CAD build for the part. Positions are in the model's coordinates, mm. A direction names the side the tool comes from. Round coordinates to 2 decimals unless told otherwise and drop trailing zeros. Loops run counter-clockwise (first coordinate to the right, second up) from the corner with the lowest first, then second, coordinate; pieces in that order, holes last. Notation, with made-up numbers: (11.5, -23.75) - (45.5, -23.75) arc R20 cw to (45.5, 5.25) - close; hole circle Ø3 at (58, 42.25). An arc over 180 degrees is marked (long way). One line per question, with ' | ' between items.
Autodesk Inventor part; units mm, degrees
ref_plane "dia1_XY" through (0, 3.175, 0) normal (1, 0, 0) x (0, 0, -1)
ref_plane "dia1_YZ" through (0, 3.175, 0) normal (0, 0, -1) x (0, 1, 0)
ref_plane "dia1_ZX" through (0, 3.175, 0) normal (0, 1, 0) x (1, 0, 0)
sketch "Sketch_1" plane through (0, 0, 0) normal (0, 0, 1) x (1, 0, 0)
  line L0 (67.5386, 0) -> (0, 0)
  line L1 (0, 0) -> (0, 3.175)
  line L2 (0, 3.175) -> (47.625, 3.175)
  line L3 (47.625, 3.175) -> (47.625, 9.6202)
  line L4 (47.625, 9.6202) -> (67.5386, 9.6202)
  line L5 (67.5386, 9.6202) -> (67.5386, 0)
  line L6 (67.5386, 0) -> (0, 0)
revolve "Revolution1" add sketch "Sketch_1" angle 360 about axis through (67.5386, 0, 0) along (1, 0, 0)
sketch "Sketch_3" plane through (0, 0, 0) normal (0, 0, 1) x (1, 0, 0)
  line L0 (0, 0) -> (-12.7, 0)
  line L1 (-12.7, 0) -> (-12.7, 2.634)
  line L2 (-12.7, 2.634) -> (-12.159, 3.175)
  line L3 (-12.159, 3.175) -> (0, 3.175)
  line L4 (0, 3.175) -> (0, 0)
  line L5 (0, 0) -> (-12.7, 0)
revolve "Revolution2" add sketch "Sketch_3" angle 360 about axis through (0, 0, 0) along (1, 0, 0)
sketch "Sketch_30" plane through (0, 0, 0) normal (0, 0, 1) x (1, 0, 0)
  line L0 (0, 0) -> (-0.254, 0)
  line L1 (-0.254, 2.921) -> (0, 2.921)
  line L2 (0, 2.921) -> (0, 3.429)
  line L3 (0, 3.429) -> (-0.254, 3.429)
  line L4 (-0.254, 3.429) -> (-0.254, 2.921)
revolve "Revolution3" cut sketch "Sketch_30" angle 360 about axis through (0, 0, 0) along (1, 0, 0)
ref_plane "dia1_XY" through (0, 3.175, 0) normal (1, 0, 0) x (0, 0, -1)
ref_plane "dia1_YZ" through (0, 3.175, 0) normal (0, 0, -1) x (0, 1, 0)
ref_plane "dia1_ZX" through (0, 3.175, 0) normal (0, 1, 0) x (1, 0, 0)
ref_plane "dia12_XY" through (0, 0, 10.2235) normal (1, 0, 0) x (0, 0, -1)
ref_plane "dia12_YZ" through (0, 0, 10.2235) normal (0, 0, -1) x (0, 1, 0)
ref_plane "dia12_ZX" through (0, 0, 10.2235) normal (0, 1, 0) x (1, 0, 0)
ref_plane "dia2_XY" through (0, -3.175, 0) normal (1, 0, 0) x (0, 0, -1)
ref_plane "dia2_YZ" through (0, -3.175, 0) normal (0, 0, -1) x (0, 1, 0)
ref_plane "dia2_ZX" through (0, -3.175, 0) normal (0, 1, 0) x (1, 0, 0)
ref_plane "dia22_XY" through (0, 0, -10.2235) normal (1, 0, 0) x (0, 0, -1)
ref_plane "dia22_YZ" through (0, 0, -10.2235) normal (0, 0, -1) x (0, 1, 0)
ref_plane "dia22_ZX" through (0, 0, -10.2235) normal (0, 1, 0) x (1, 0, 0)
ref_plane "rl1_XY" through (-12.7, 0, 0) normal (1, 0, 0) x (0, 0, -1)
ref_plane "rl1_YZ" through (-12.7, 0, 0) normal (0, 0, -1) x (0, 1, 0)
ref_plane "rl1_ZX" through (-12.7, 0, 0) normal (0, 1, 0) x (1, 0, 0)
ref_plane "rl2_XY" through (0, 0, 0) normal (1, 0, 0) x (0, 0, -1)
ref_plane "rl2_YZ" through (0, 0, 0) normal (0, 0, -1) x (0, 1, 0)
ref_plane "rl2_ZX" through (0, 0, 0) normal (0, 1, 0) x (1, 0, 0)
ref_plane "rod_cp_XY" through (0, 0, 0) normal (1, 0, 0) x (0, 0, -1)
ref_plane "rod_cp_YZ" through (0, 0, 0) normal (0, 0, -1) x (0, 1, 0)
ref_plane "rod_cp_ZX" through (0, 0, 0) normal (0, 1, 0) x (1, 0, 0)
ref_plane "thd1_XY" through (-12.7, 3.175, 0) normal (1, 0, 0) x (0, 0, -1)
ref_plane "thd1_YZ" through (-12.7, 3.175, 0) normal (0, 0, -1) x (0, 1, 0)
ref_plane "thd1_ZX" through (-12.7, 3.175, 0) normal (0, 1, 0) x (1, 0, 0)
ref_plane "thd2_XY" through (-12.7, -3.175, 0) normal (1, 0, 0) x (0, 0, -1)
ref_plane "thd2_YZ" through (-12.7, -3.175, 0) normal (0, 0, -1) x (0, 1, 0)
ref_plane "thd2_ZX" through (-12.7, -3.175, 0) normal (0, 1, 0) x (1, 0, 0)
ref_plane "to_rod_clevis_XY" through (-16.764, 0, 0) normal (1, 0, 0) x (0, 0, -1)
ref_plane "to_rod_clevis_YZ" through (-16.764, 0, 0) normal (0, 0, -1) x (0, 1, 0)
ref_plane "to_rod_clevis_ZX" through (-16.764, 0, 0) normal (0, 1, 0) x (1, 0, 0)
properties part number "C-0410000_rod"
(1) Drop flat-ended pins along their axis: P1, Ø8, axis at x = 46, y = 5, coming from the +Z side; P2, Ø1.5, axis at y = 4.5, z = -3.5, coming from the -X side (3 decimals); P3, Ø10, axis at x = -4.5, y = -5.5, coming from the +Z side. Give the stop position or say it passes through.
Results found:
P1: stops at z = 9.53 | P2: stops at x = 47.625 | P3: stops at z = 3.14
(2) Cut at C-C, the plane x = 49. Write the cut outline in (y, z).
Results found:
outline: circle Ø19.24 at (0, 0)
(3) Cut at A-A, the plane z = 0. Write the cut outline in (x, y) (3 decimals).
Results found:
outline: (-12.7, -2.634) - (-12.159, -3.175) - (-0.254, -3.175) - (-0.254, -2.921) - (0, -2.921) - (0, -3.175) - (47.625, -3.175) - (47.625, -9.62) - (67.539, -9.62) - (67.539, 9.62) - (47.625, 9.62) - (47.625, 3.175) - (0, 3.175) - (0, 2.921) - (-0.254, 2.921) - (-0.254, 3.175) - (-12.159, 3.175) - (-12.7, 2.634) - close
(4) Cut at D-D, the plane x = 31. Write the cut outline in (y, z) (3 decimals).
Results found:
outline: circle Ø6.35 at (0, 0)
(5) Tool access for faces 1 (the face through (24.15, -0.69, -3.1)), 2 (the face through (-12.7, 0, 0)): list every direction of +Z, -Z, +X, -X, +Y, -Y with a clear straight run to the whole face (end or side of a thin tool).
Results found:
face 1: -X | face 2: +Z, -Z, -X, +Y, -Y
(6) Probe L1, parallel to X at y = -0.5, z = 7.5 (3 decimals); L2, parallel to Z at x = 50, y = 0.25; L3, parallel to Z at x = 26, y = -1.25. List the from-to ranges inside material, lowest first.
Results found:
L1: x = 47.625 to 67.539 | L2: z = -9.62 to 9.62 | L3: z = -2.92 to 2.92
